Could you check a few things on this model? Use its own coordinates, in mm. Face numbers are marked on the shaded views. A direction names the side the tool comes from. Coordinates: 2 decimals unless noted, no trailing zeros. Write each loop counter-clockwise with the first axis right and the second up, starting at its lowest first coordinate (ties: lowest second). Pieces come first, ordered by that corner, then holes.
```python
from build123d import *
from build123d.topology import SkipClean

# Parameters (mm, degrees)
BASEBODY_DEPTH           = 2
SKETCH_2_R               = 5.9
FRONTBODY_DEPTH          = 1.5
SOCKET_START             = -1.5
SOCKET_DEPTH             = 1.5
SKETCH_3_3_R             = 0.75
SOCKETPINS_DEPTH         = 1.5
SKETCH_4_R               = 5
RBODY_DEPTH              = 4.8
SKETCH_5_R               = 1.4
HOLE1_DEPTH              = 2
SKETCH_5_3_R             = 1
HOLE2_DEPTH              = 16.792798992
LIGHTING_START           = -6
LIGHTING_DEPTH           = 6
SKETCH_7_R               = 5
RBODY2_DEPTH             = 1
LIGHTING3_DEPTH          = 17.248461466
LIGHTING3_DEPTH_BACK     = 17.248461466
SKETCH_8_W               = 3.4
SKETCH_8_H               = 2
CUT_EXTRUDE_8_DEPTH      = 17.248461466
CUT_EXTRUDE_8_DEPTH_BACK = 17.248461466
SKETCH_9_W               = 5.8
SKETCH_9_H               = 2
SKETCH_10_W              = 5.7
SKETCH_10_H              = 1
EXTRUDE_2_DEPTH          = 4
EXTRUDE_3_DEPTH          = 10.2
SKETCH_11_R              = 0.9
EXTRUDE_4_DEPTH          = 4.4
EXTRUDE_5_DEPTH          = 8.3


# Read off the part's stored shape, not the designer's step: Socket
with BuildPart() as part:
    # Эскиз1 → BaseBody (new body)
    with BuildSketch(Plane.XY):
        with BuildLine():
            Line((-10.715789474, 2.742600218), (-2.776052632, 6.262270498))
            ThreePointArc((-2.776052632, 6.262270498), (0, 6.85), (2.776052632, 6.262270498))
            Line((2.776052632, 6.262270498), (10.715789474, 2.742600218))
            ThreePointArc((10.715789474, 2.742600218), (12.5, 0), (10.715789474, -2.742600218))
            Line((10.715789474, -2.742600218), (2.776052632, -6.262270498))
            ThreePointArc((2.776052632, -6.262270498), (0, -6.85), (-2.776052632, -6.262270498))
            Line((-2.776052632, -6.262270498), (-10.715789474, -2.742600218))
            ThreePointArc((-10.715789474, -2.742600218), (-12.5, 0), (-10.715789474, 2.742600218))
        make_face()
    extrude(amount=BASEBODY_DEPTH)

    # Эскиз2 → FrontBody (add)
    with BuildSketch(Plane(origin=(0, 0, 0), x_dir=(-1, 0, 0), z_dir=(0, 0, -1))):
        Circle(SKETCH_2_R)
    extrude(amount=FRONTBODY_DEPTH)

    # Socket outline → Socket (cut)
    with BuildSketch(Plane(origin=(0, 0, -1.5), x_dir=(-1, 0, 0), z_dir=(0, 0, -1)).offset(SOCKET_START)):
        with BuildLine():
            Line((-2, 4.85412196), (-2, 4.363484846))
            ThreePointArc((-2, 4.363484846), (0, -4.8), (2, 4.363484846))
            Line((2, 4.363484846), (2, 4.85412196))
            ThreePointArc((2, 4.85412196), (0, 5.25), (-2, 4.85412196))
        make_face()
        with BuildLine():
            ThreePointArc((-3.567912555, -2.4), (-3.947776364, 1.704424179), (-0.7, 4.242640687))
            Line((-0.7, 4.242640687), (-0.7, 3.542640687))
            Line((-0.7, 3.542640687), (0.7, 3.542640687))
            Line((0.7, 3.542640687), (0.7, 4.242640687))
            ThreePointArc((0.7, 4.242640687), (3.947776364, 1.704424179), (3.567912555, -2.4))
            Line((3.567912555, -2.4), (2.5, -2.4))
            Line((2.5, -2.4), (2.5, -3.498571137))
            ThreePointArc((2.5, -3.498571137), (0, -4.3), (-2.5, -3.498571137))
            Line((-2.5, -3.498571137), (-2.5, -2.4))
            Line((-2.5, -2.4), (-3.567912555, -2.4))
        make_face(mode=Mode.SUBTRACT)
    extrude(amount=SOCKET_DEPTH, mode=Mode.SUBTRACT)

    # Эскиз3<3> → SocketPins (cut)
    with BuildSketch(Plane(origin=(0, 0, -1.5), x_dir=(-1, 0, 0), z_dir=(0, 0, -1))):
        with Locations((-2, 1.6)):
            Circle(SKETCH_3_3_R)
        with Locations((-2.5, -0.4)):
            Circle(SKETCH_3_3_R)
        with Locations((-1, -2.4)):
            Circle(SKETCH_3_3_R)
        with Locations((1, -2.4)):
            Circle(SKETCH_3_3_R)
        with Locations((2.5, -0.4)):
            Circle(SKETCH_3_3_R)
        with Locations((2, 1.6)):
            Circle(SKETCH_3_3_R)
    extrude(amount=-SOCKETPINS_DEPTH, mode=Mode.SUBTRACT)

    # Эскиз4 → RBody (add)
    with SkipClean():  # the faces are left unmerged after this step: merging them gives an invalid solid
        with BuildSketch(Plane.XY.offset(2)):
            with BuildLine():
                ThreePointArc((-6.5, 0), (-7.378679656, 2.121320344), (-9.5, 3))
                ThreePointArc((-9.5, 3), (-10.121369192, 2.934944689), (-10.715789474, 2.742600218))
                ThreePointArc((-10.715789474, 2.742600218), (-12.5, 0), (-10.715789474, -2.742600218))
                ThreePointArc((-10.715789474, -2.742600218), (-10.121369192, -2.934944689), (-9.5, -3))
                ThreePointArc((-9.5, -3), (-7.378679656, -2.121320344), (-6.5, 0))
            make_face()
            with BuildLine():
                Line((-4, 3), (-9.5, 3))
                ThreePointArc((-9.5, 3), (-7.378679656, 2.121320344), (-6.5, 0))
                ThreePointArc((-6.5, 0), (-7.378679656, -2.121320344), (-9.5, -3))
                Line((-9.5, -3), (-4, -3))
                ThreePointArc((-4, -3), (-5, 0), (-4, 3))
            make_face()
            Circle(SKETCH_4_R)
            with BuildLine():
                Line((9.5, 3), (4, 3))
                ThreePointArc((4, 3), (4.74341649, 1.58113883), (5, 0))
                ThreePointArc((5, 0), (4.74341649, -1.58113883), (4, -3))
                Line((4, -3), (9.5, -3))
                ThreePointArc((9.5, -3), (6.5, 0), (9.5, 3))
            make_face()
            with BuildLine():
                ThreePointArc((10.715789474, 2.742600218), (10.121369192, 2.934944689), (9.5, 3))
                ThreePointArc((9.5, 3), (6.5, 0), (9.5, -3))
                ThreePointArc((9.5, -3), (10.121369192, -2.934944689), (10.715789474, -2.742600218))
                ThreePointArc((10.715789474, -2.742600218), (12.014693661, -1.635944923), (12.5, 0))
                ThreePointArc((12.5, 0), (12.014693661, 1.635944923), (10.715789474, 2.742600218))
            make_face()
        extrude(amount=RBODY_DEPTH)

    # Эскиз5 → Hole1 (cut)
    with SkipClean():  # the faces are left unmerged after this step: merging them gives an invalid solid
        with BuildSketch(Plane(origin=(0, 0, 0), x_dir=(-1, 0, 0), z_dir=(0, 0, -1))):
            with Locations((9.5, 0)):
                Circle(SKETCH_5_R)
            with Locations((-9.5, 0)):
                Circle(SKETCH_5_R)
        extrude(amount=-HOLE1_DEPTH, mode=Mode.SUBTRACT)

    # Эскиз5<3> → Hole2 (cut, through all)
    with SkipClean():  # the faces are left unmerged after this step: merging them gives an invalid solid
        with BuildSketch(Plane(origin=(0, 0, 0), x_dir=(-1, 0, 0), z_dir=(0, 0, -1))):
            with Locations((9.5, 0)):
                Circle(SKETCH_5_3_R)
            with Locations((-9.5, 0)):
                Circle(SKETCH_5_3_R)
        extrude(amount=-HOLE2_DEPTH, mode=Mode.SUBTRACT)

    # Эскиз6 → Lighting (cut)
    with SkipClean():  # the faces are left unmerged after this step: merging them gives an invalid solid
        with BuildSketch(Plane.XY.offset(6.8).offset(LIGHTING_START)):
            with BuildLine():
                Line((-7.7, 2.4), (-4.38634244, 2.4))
                ThreePointArc((-4.38634244, 2.4), (-5, 0), (-4.38634244, -2.4))
                Line((-4.38634244, -2.4), (-7.7, -2.4))
                ThreePointArc((-7.7, -2.4), (-6.5, 0), (-7.7, 2.4))
            make_face()
        lighting = extrude(amount=LIGHTING_DEPTH, mode=Mode.SUBTRACT)

    # Lighting2: Lighting across plane
    with SkipClean():  # the faces are left unmerged after this step: merging them gives an invalid solid
        add(lighting.mirror(Plane(origin=(0, 0, 0), x_dir=(0, 0, 1), z_dir=(1, 0, 0))), mode=Mode.SUBTRACT)

    # Эскиз7 → RBody2 (add)
    with SkipClean():  # the faces are left unmerged after this step: merging them gives an invalid solid
        with BuildSketch(Plane.XY.offset(6.8)):
            with Locations(Location((0, 0, 0), (0, 0, 151.314597986))):
                Circle(SKETCH_7_R)
        extrude(amount=RBODY2_DEPTH)

    # Эскиз8 → Lighting3 (cut, two sides: drawn at the far end of the back side and taken through both)
    with SkipClean():  # the faces are left unmerged after this step: merging them gives an invalid solid
        with BuildSketch(Plane(origin=(0, 0, 0), x_dir=(0, 0, -1), z_dir=(1, 0, 0)).offset(-LIGHTING3_DEPTH_BACK)):
            with Locations((-6.1, -4)):
                Rectangle(SKETCH_8_W, SKETCH_8_H)
        extrude(amount=LIGHTING3_DEPTH + LIGHTING3_DEPTH_BACK, mode=Mode.SUBTRACT)

    # Эскиз9 → Вырез-Вытянуть8 (cut, two sides: drawn at the far end of the back side and taken through both)
    with SkipClean():  # the faces are left unmerged after this step: merging them gives an invalid solid
        with BuildSketch(Plane(origin=(0, 0, 0), x_dir=(0, 0, -1), z_dir=(1, 0, 0)).offset(-CUT_EXTRUDE_8_DEPTH_BACK)):
            with Locations((-4.9, 4)):
                Rectangle(SKETCH_9_W, SKETCH_9_H)
        extrude(amount=CUT_EXTRUDE_8_DEPTH + CUT_EXTRUDE_8_DEPTH_BACK, mode=Mode.SUBTRACT)

    # Эскиз10 → Бобышка-Вытянуть2 (add)
    with SkipClean():  # the faces are left unmerged after this step: merging them gives an invalid solid
        with BuildSketch(Plane.XY.offset(2)):
            with Locations((0, 3.5)):
                Rectangle(SKETCH_10_W, SKETCH_10_H)
        extrude(amount=EXTRUDE_2_DEPTH)

    # Эскиз10<3> → Бобышка-Вытянуть3 (add)
    with SkipClean():  # the faces are left unmerged after this step: merging them gives an invalid solid
        with BuildSketch(Plane.XY.offset(2)):
            Polygon((-4.5, 4), (-2.85, 4), (2.85, 4), (4.5, 4), (4.5, 5), (-4.5, 5), align=None)
        extrude(amount=EXTRUDE_3_DEPTH)

    # Эскиз11 → Бобышка-Вытянуть4 (add)
    with SkipClean():  # the faces are left unmerged after this step: merging them gives an invalid solid
        with BuildSketch(Plane.XY.offset(7.8)):
            with Locations((-3.4, -2)):
                Circle(SKETCH_11_R)
            with Locations((3.4, -2)):
                Circle(SKETCH_11_R)
        extrude(amount=EXTRUDE_4_DEPTH)

    # Эскиз12 → Бобышка-Вытянуть5 (add)
    with SkipClean():  # the faces are left unmerged after this step: merging them gives an invalid solid
        with BuildSketch(Plane.XY.offset(7.8)):
            Polygon((1.63, -1.4), (1.63, -2.1), (2.37, -2.1), (2.37, -1.4), (2.22, -1.4), (2.22, -1.9), (1.78, -1.9), (1.78, -1.4), align=None)
            Polygon((2.832000989, -0.445092269), (3.532000989, -0.445092269), (3.532000989, 0.294907731), (2.832000989, 0.294907731), (2.832000989, 0.144907731), (3.332000989, 0.144907731), (3.332000989, -0.295092269), (2.832000989, -0.295092269), align=None)
            Polygon((2.552578831, 1.441994282), (3.252578831, 1.441994282), (3.252578831, 2.181994282), (2.552578831, 2.181994282), (2.552578831, 2.031994282), (3.052578831, 2.031994282), (3.052578831, 1.591994282), (2.552578831, 1.591994282), align=None)
        extrude_5 = extrude(amount=EXTRUDE_5_DEPTH)

    # Зеркальное отражение3: Бобышка-Вытянуть5 across plane
    with SkipClean():  # the faces are left unmerged after this step: merging them gives an invalid solid
        add(extrude_5.mirror(Plane(origin=(0, 0, 0), x_dir=(0, 0, 1), z_dir=(1, 0, 0))))


solid = part.part
```
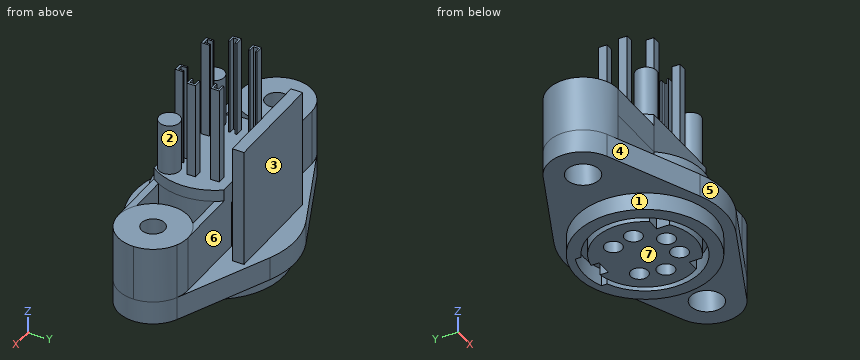
1. For pin 1 (0.8 mm diameter, centred on y = 4, z = -1, fed in from -X); pin 2 (5 mm diameter, centred on x = 1, y = 1.5, fed in from +Z); pin 3 (2 mm diameter, centred on y = 0, z = 10, fed in from +X); pin 4 (0.8 mm diameter, centred on x = 9, y = 0, fed in from -Z), each with a flat end and sliding along its axis, tell me the tip position at first contact or that it passes through.
Verdict:
pin 1: stops at x = -4.67
pin 2: stops at z = 16.1
pin 3: stops at x = 3.53
pin 4: passes through
2. I want a section at A-A on z = 3. Please give me the cut outline in (x, y), plus the area to 3 significant figures.
Verdict:
outline: (-9.5, -3) - (-4, -3) arc R5 ccw to (4, -3) - (9.5, -3) arc R3 ccw to (9.5, 3) - (2.85, 3) - (2.85, 4) - (4.5, 4) - (4.5, 5) - (-4.5, 5) - (-4.5, 4) - (-2.85, 4) - (-2.85, 3) - (-9.5, 3) arc R3 ccw to start; hole circle Ø2 at (-9.5, 0); hole (-7.7, -2.4) - (-4.39, -2.4) arc R5 cw to (-4.39, 2.4) - (-7.7, 2.4) arc R3 cw to start; hole (4.39, -2.4) - (7.7, -2.4) arc R3 cw to (7.7, 2.4) - (4.39, 2.4) arc R5 cw to start; hole circle Ø2 at (9.5, 0)
area: 142 mm2
3. On a 3-axis mill with a long thin cutter (end or side, diameter ignored), from which of +Z, -Z, +X, -X, +Y, -Y can I reach the whole of each face in a straight line? I mean the marked faces 1, 2, 3 and 4. Say none if no direction works.
Verdict:
face 1: -Z
face 2: +Z
face 3: +Z, +X, -X, +Y
face 4: +Z, -Z, -X, -Y
4. I want a section at B-B on z = 14.25. Give the number of separate pieces and of enclosed holes in the cut face, plus the area to 3 significant figures.
Verdict:
separate pieces: 6
enclosed holes: 0
area: 1.79 mm2
5. Please list where these lines run through material, in increasing order: line 1 along Y through (x, z) = (-7, 1.5); line 2 along Z through (x, y) = (2.25, 2); line 3 along Z through (x, y) = (1.5, 2.25).
Verdict:
line 1: y = -4.39 to -2.4, -1.66 to 1.66, 2.4 to 4.39
line 2: z = 0 to 7.8
line 3: z = -1.5 to 7.8
6. If we mould it in two halves opening along Y, with no side actions, what happens to the marked faces 5, 6 and 7? For each: pulls with the +Y half, pulls with the -Y half, needs draft (parallel to the pull), parting line crosses it, or undercut.
Verdict:
face 5: pulls with the -Y half
face 6: undercut
face 7: needs draft
